```python
from build123d import *

# Parameters (mm, degrees)
F0_R     = 30
F1_DEPTH = 39
F2_R     = 15
F3_DEPTH = 39.001
F4_SIZE  = 1
F5_R     = 24.743506
F5_R_2   = 19.921836
F6_DEPTH = 1
F7_R     = 24.743506
F7_R_2   = 19.921836
F8_DEPTH = 1


with BuildPart() as f1:
    # F0 (on Front) → F1 (new body)
    with BuildSketch(Plane.XZ):
        Circle(F0_R)
    extrude(amount=F1_DEPTH)

    # F2 (on face) → F3 (cut, through all)
    with BuildSketch(Plane.XZ.offset(39)):
        Circle(F2_R)
    extrude(amount=-F3_DEPTH, mode=Mode.SUBTRACT)

    # F4
    f4_edges = [f1.edges().sort_by_distance(p)[0] for p in [
        (-30, -39, 0),
        (-15, -39, 0),
        (-30, 0, 0),
        (-15, 0, 0),
    ]]
    chamfer(f4_edges, length=F4_SIZE)

    # F5 (on face) → F6 (cut)
    with BuildSketch(Plane(origin=(0, 0, 0), x_dir=(-1, 0, 0), z_dir=(0, 1, 0))):
        Circle(F5_R)
        Circle(F5_R_2, mode=Mode.SUBTRACT)
    extrude(amount=-F6_DEPTH, mode=Mode.SUBTRACT)

    # F7 (on face) → F8 (cut)
    with BuildSketch(Plane.XZ.offset(39)):
        Circle(F7_R)
        Circle(F7_R_2, mode=Mode.SUBTRACT)
    extrude(amount=-F8_DEPTH, mode=Mode.SUBTRACT)


solid = f1.part
```
Can you work these out from the model? Positions are in its coordinate system, mm. A direction names the side the tool comes from. Round coordinates to 2 decimals unless told otherwise and drop trailing zeros. Loops run counter-clockwise (first coordinate to the right, second up) from the corner with the lowest first, then second, coordinate; pieces in that order, holes last. Notation, with made-up numbers: M 9.25,15.25 L 36.25,15.25 A24 ccw 36.25,30.25 Z; hole C 32.5,50 d10. An arc over 180 degrees is marked long. Answer as a JSON object with one key per item and string values. Group by question number.
Q1. On a 3-axis mill with a long thin cutter (end or side, diameter ignored), from which of +Z, -Z, +X, -X, +Y, -Y can I reach the whole of each face in a straight line? I mean faces 5 (the flat face through (-17, -38, 11)), 6 (the flat face through (-0.1, 0, 16.3)), 7 (the cylindrical face through (-23.6, -0.49, 7.43)). Say none if no direction works.
Q2. Will these pins go through, and if not, where does the flat tip stop? pin 1 (12 mm diameter, centred on x = 0, y = -22, fed in from +Z); pin 2 (6 mm diameter, centred on x = 22, y = -12, fed in from -Z); pin 3 (6 mm diameter, centred on y = -23, z = 15, fed in from -X).
Q3. Please list where these lines run through material, in increasing order: L1, parallel to Z at x = 0, y = -38.45; L2, parallel to Z at x = -11, y = -12.5; L3, parallel to Z at x = 0, y = -0.3.
Q4. We'd pull the mould along Z, two halves only. Please class faces 1 (the cylindrical face through (23.6, -38.51, 7.43)), 2 (the cylindrical face through (19.002, -38.507, 5.984)), 3 (the cylindrical face through (-29.97, -19.24, 1.32)), 4 (the flat face through (-0.1, -39, 16.3)): +Z half, -Z half, draft (parallel to the pull), parting line (faces both ways), or undercut.
Q5. Imagine slicing it at C-C, the plane y = -27. Please give me the cut outline in (x, z).
Findings:
{
 "1": {"face 5": "-Y", "face 6": "+Z, -Z, +X, -X, +Y", "face 7": "+Y"},
 "2": {"pin 1": "stops at z = 30", "pin 2": "stops at z = -23.22", "pin 3": "stops at x = -27.5"},
 "3": {"L1": "z = -29.55 to -24.74, -19.92 to -15.45, 15.45 to 19.92, 24.74 to 29.55", "L2": "z = -27.91 to -10.2, 10.2 to 27.91", "L3": "z = -29.3 to -24.74, -19.92 to -15.7, 15.7 to 19.92, 24.74 to 29.3"},
 "4": {"face 1": "undercut", "face 2": "undercut", "face 3": "parting line", "face 4": "draft"},
 "5": {"outline": "C 0,0 d60; hole C 0,0 d30"}
}
